Autodesk Fusion 360 part; units mm, degrees
sketch "Sketch1" plane through (0, 0, 0) normal (0, 0, 1) x (1, 0, 0)
  line L0 (-120.55, 25.4) -> (120.65, 25.4)
  line L1 (120.65, 25.4) -> (120.65, -25.4)
  line L2 (120.65, -25.4) -> (-120.55, -25.4)
  line L3 (-120.55, -25.4) -> (-120.55, 25.4)
  dimension "d3" = 241.2
  dimension "d4" = 50.8
  dimension "d5" = 25.4
  dimension "d6" = 120.65
extrude "Extrude1" add sketch "Sketch1" along normal blind 2.5
sketch "Sketch2" plane through (0, 0, 2.5) normal (0, 0, 1) x (-1, 0, 0)
  line L0 (120.55, 25.4) -> (-120.65, 25.4)
  line L1 (-120.65, 25.4) -> (-120.65, -25.4)
  line L2 (-120.65, -25.4) -> (120.55, -25.4)
  line L3 (120.55, -25.4) -> (120.55, 25.4)
  line L4 (13.4, -15.4) -> (-13.4, -15.4)
  line L5 (-15.4, -13.4) -> (-15.4, 13.4)
  line L6 (-13.4, 15.4) -> (13.4, 15.4)
  line L7 (15.4, 13.4) -> (15.4, -13.4)
  arc A0 (13.4, -15.4) -> (15.4, -13.4) centre (13.4, -13.4) ccw
  arc A1 (-15.4, -13.4) -> (-13.4, -15.4) centre (-13.4, -13.4) ccw
  arc A2 (-13.4, 15.4) -> (-15.4, 13.4) centre (-13.4, 13.4) ccw
  arc A3 (15.4, 13.4) -> (13.4, 15.4) centre (13.4, 13.4) ccw
  dimension "d7" = 30.8
  dimension "d8" = 30.8
  dimension "d9" = 15.4
  dimension "d10" = 15.4
  dimension "d11" = 2
extrude "Extrude2" cut sketch "Sketch2" against normal blind 2.5 contours L4 L5 L6 L7 A0 A1 A2 A3
sketch "Sketch4" plane through (0, 0, 2.5) normal (0, 0, 1) x (-1, 0, 0)
  line L0 (15.4, 13.4) -> (15.4, -13.4)
  arc A0 (13.4, -15.4) -> (15.4, -13.4) centre (13.4, -13.4) ccw
  line L1 (13.4, -15.4) -> (-13.4, -15.4)
  arc A1 (-15.4, -13.4) -> (-13.4, -15.4) centre (-13.4, -13.4) ccw
  line L2 (-15.4, -13.4) -> (-15.4, 13.4)
  arc A2 (-13.4, 15.4) -> (-15.4, 13.4) centre (-13.4, 13.4) ccw
  line L3 (-13.4, 15.4) -> (13.4, 15.4)
  arc A3 (15.4, 13.4) -> (13.4, 15.4) centre (13.4, 13.4) ccw
  line L4 (120.55, 25.4) -> (-120.65, 25.4)
  line L5 (-120.65, 25.4) -> (-120.65, -25.4)
  line L6 (-120.65, -25.4) -> (120.55, -25.4)
  line L7 (120.55, -25.4) -> (120.55, 25.4)
  line L8 (18, -20) -> (-18, -20)
  line L9 (-20, -18) -> (-20, 18)
  line L10 (-18, 20) -> (18, 20)
  line L11 (20, 18) -> (20, -18)
  arc A4 (18, -20) -> (20, -18) centre (18, -18) ccw
  arc A5 (-20, -18) -> (-18, -20) centre (-18, -18) ccw
  arc A6 (-18, 20) -> (-20, 18) centre (-18, 18) ccw
  arc A7 (20, 18) -> (18, 20) centre (18, 18) ccw
  dimension "d18" = 40
  dimension "d19" = 40
  dimension "d20" = 20
  dimension "d21" = 20
  dimension "d22" = 2
extrude "Extrude3" add sketch "Sketch4" along normal blind 2.5 contours L8 L9 L10 L11 A4 A5 A6 A7
sketch "Sketch6" plane through (0, 0, 5) normal (0, 0, 1) x (-1, 0, 0)
  arc A0 (13.4, -15.4) -> (15.4, -13.4) centre (13.4, -13.4) ccw
  line L0 (13.4, -15.4) -> (-13.4, -15.4)
  arc A1 (-15.4, -13.4) -> (-13.4, -15.4) centre (-13.4, -13.4) ccw
  line L1 (-15.4, -13.4) -> (-15.4, 13.4)
  arc A2 (-13.4, 15.4) -> (-15.4, 13.4) centre (-13.4, 13.4) ccw
  line L2 (-13.4, 15.4) -> (13.4, 15.4)
  arc A3 (15.4, 13.4) -> (13.4, 15.4) centre (13.4, 13.4) ccw
  line L3 (15.4, 13.4) -> (15.4, -13.4)
  arc A4 (18, -20) -> (20, -18) centre (18, -18) ccw
  line L4 (20, -18) -> (20, 18)
  arc A5 (20, 18) -> (18, 20) centre (18, 18) ccw
  line L5 (18, 20) -> (-18, 20)
  arc A6 (-18, 20) -> (-20, 18) centre (-18, 18) ccw
  line L6 (-20, 18) -> (-20, -18)
  arc A7 (-20, -18) -> (-18, -20) centre (-18, -18) ccw
  line L7 (-18, -20) -> (18, -20)
  point P0 (17, -17)
  point P1 (-17, -17)
  point P2 (-17, 17)
  point P3 (17, 17)
  dimension "d29" = 34
  dimension "d30" = 34
  dimension "d31" = 17
  dimension "d32" = 17
hole "Hole1" at (-17, 17, 5) at (17, 17, 5) at (17, -17, 5) at (-17, -17, 5) direction (0, 0, -1) diameter 2.54 depth 5 tip angle 118
chamfer "Chamfer1" distance 2.5 distance2 2.5 8 edges at (0, -20, 2.5) (-19.4142, -19.4142, 2.5) (-20, 0, 2.5) (-19.4142, 19.4142, 2.5) (0, 20, 2.5) (19.4142, 19.4142, 2.5) (20, 0, 2.5) (19.4142, -19.4142, 2.5) measured on face at (87.1, -6, 2.5) measured on face at (87.1, -6, 2.5) measured on face at (87.1, -6, 2.5) measured on face at (87.1, -6, 2.5) measured on face at (87.1, -6, 2.5) measured on face at (87.1, -6, 2.5) measured on face at (87.1, -6, 2.5) measured on face at (87.1, -6, 2.5)
fillet "Fillet1" radius 2.5 8 edges at (22.5, 0, 2.5) (21.182, 21.182, 2.5) (0, 22.5, 2.5) (-21.182, 21.182, 2.5) (-22.5, 0, 2.5) (-21.182, -21.182, 2.5) (0, -22.5, 2.5) (21.182, -21.182, 2.5)
sketch "Sketch7" plane through (0, 0, 0) normal (0, 0, -1) x (1, 0, 0)
  circle A0 centre (17, 17) radius 1.27
  circle A1 centre (-17, -17) radius 1.27
  circle A2 centre (17, -17) radius 1.27
  circle A3 centre (-17, 17) radius 1.27
  line L0 (-15.4, -13.4) -> (-15.4, 13.4)
  arc A4 (-13.4, 15.4) -> (-15.4, 13.4) centre (-13.4, 13.4) ccw
  line L1 (-13.4, 15.4) -> (13.4, 15.4)
  arc A5 (15.4, 13.4) -> (13.4, 15.4) centre (13.4, 13.4) ccw
  line L2 (15.4, 13.4) -> (15.4, -13.4)
  arc A6 (13.4, -15.4) -> (15.4, -13.4) centre (13.4, -13.4) ccw
  line L3 (13.4, -15.4) -> (-13.4, -15.4)
  arc A7 (-15.4, -13.4) -> (-13.4, -15.4) centre (-13.4, -13.4) ccw
  line L4 (120.65, 25.4) -> (-120.55, 25.4)
  line L5 (-120.55, 25.4) -> (-120.55, -25.4)
  line L6 (-120.55, -25.4) -> (120.65, -25.4)
  line L7 (120.65, -25.4) -> (120.65, 25.4)
  point P0 (-112.9, 15)
  point P1 (-112.9, -15)
  point P2 (113, 15)
  point P3 (113, -15)
  dimension "d40" = 30
  dimension "d41" = 7.65
  dimension "d42" = 7.65
  dimension "d48" = 10.4
hole "Hole2" at (-112.9, -15, 0) at (-112.9, 15, 0) at (113, -15, 0) at (113, 15, 0) direction (0, 0, 1) diameter 4.5 depth 5 tip angle 180 countersink diameter 9.4 countersink angle 90
extrude "Extrude5" add 1 faces at (-17.0425, 4.4667, 5) along direction (0, 0, 1) blind 10
equation "d3 = 9.5 in - 0.1 mm"
equation "d6 = ( 9.5 / 2 ) * 1 in"
equation "d41 = ( ( 15.4 / 2 ) * 1 mm ) - 0.05 * 1 mm"
equation "d42 = ( ( 15.4 / 2 ) * 1 mm ) - 0.05 * 1 mm"
equation "d48 = ( 2 in - 30 mm ) / 2"
Input: part model. Units: mm. Frame: model coordinates. A direction names the side the tool comes from. Give positions to 0.01 mm unless a question says otherwise; leave off trailing zeros. Write each loop counter-clockwise with the first axis right and the second up, starting at its lowest first coordinate (ties: lowest second). Pieces come first, ordered by that corner, then holes. Notation, with made-up numbers: (-6, 74.5) - (27, 74.5) arc R16 ccw to (27, 82.5) - close; hole circle Ø1 at (13.25, -33). An arc over 180 degrees is marked (long way). Write item = value, one per line. Start each with the question number.
1) Cut plane D-D (x = -42). Return loops of the section in (y, z).
2) Reachability of faces 4 (the face through (20, 0, 10)), 5 (the face through (0, -20, 10)), 6 (the face through (0, 15.4, 7)) from +Z, -Z, +X, -X, +Y, -Y: full face, straight path, thin tool, end or side. Return the list, or none.
3) Draft query along X for faces 1 (the face through (-20, 0, 10)), 2 (the face through (0, 20, 10)), 3 (the face through (-15.4, 0, 7)). Return one class per face: pulls with the +X half, pulls with the -X half, needs draft (parallel to the pull), parting line crosses it, or undercut.
4) Cut plane C-C (y = -3). Return loops of the section in (x, z).
5) Cut plane A-A (x = -112.9). Return loops of the section in (y, z), and give its area (3 significant figures).
6) Material intervals for L1, parallel to X at y = -17, z = 8; L2, parallel to Y at x = -4, z = 6.5, sorted ascending. Write a range as [from, to].
7) Cut plane B-B (z = 8.5). Return loops of the section in (x, y), and give its area (3 significant figures).
8) Pin query (flat end, axial travel): pin 1 (4 mm diameter, centred on x = -17, y = 17, fed in from +Z); pin 2 (5 mm diameter, centred on x = -8.5, z = 9, fed in from -Y); pin 3 (5 mm diameter, centred on x = -112.9, y = -15, fed in from -Z); pin 4 (1.5 mm diameter, centred on y = -12, z = 5, fed in from +X). Return the tip coordinate at first contact, or that it passes through.
Answers follow:
q1.outline = (-25.4, 0) - (25.4, 0) - (25.4, 2.5) - (-25.4, 2.5) - close
q2.face_4 = +Z, +X, +Y, -Y
q2.face_5 = +Z, +X, -X, -Y
q2.face_6 = +Z, -Z
q3.face_1 = pulls with the -X half
q3.face_2 = needs draft
q3.face_3 = undercut
q4.outline = (-120.55, 0) - (-15.4, 0) - (-15.4, 15) - (-20, 15) - (-20, 5) - (-21.77, 3.23) arc R2.5 cw to (-23.54, 2.5) - (-120.55, 2.5) - close; (15.4, 0) - (120.65, 0) - (120.65, 2.5) - (23.54, 2.5) arc R2.5 cw to (21.77, 3.23) - (20, 5) - (20, 15) - (15.4, 15) - close
q5.outline = (-25.4, 0) - (-19.7, 0) - (-17.25, 2.45) - (-17.25, 2.5) - (-25.4, 2.5) - close; (-12.75, 2.45) - (-10.3, 0) - (10.3, 0) - (12.75, 2.45) - (12.75, 2.5) - (-12.75, 2.5) - close; (17.25, 2.45) - (19.7, 0) - (25.4, 0) - (25.4, 2.5) - (17.25, 2.5) - close
q5.area = 92.5 mm^2
q6.L1 = [-20, -18.27], [-15.73, 15.73], [18.27, 20]
q6.L2 = [-20, -15.4], [15.4, 20]
q7.outline = (-20, -18) arc R2 ccw to (-18, -20) - (18, -20) arc R2 ccw to (20, -18) - (20, 18) arc R2 ccw to (18, 20) - (-18, 20) arc R2 ccw to (-20, 18) - close; hole circle Ø2.54 at (-17, -17); hole circle Ø2.54 at (-17, 17); hole (-15.4, -13.4) arc R2 ccw to (-13.4, -15.4) - (13.4, -15.4) arc R2 ccw to (15.4, -13.4) - (15.4, 13.4) arc R2 ccw to (13.4, 15.4) - (-13.4, 15.4) arc R2 ccw to (-15.4, 13.4) - close; hole circle Ø2.54 at (17, -17); hole circle Ø2.54 at (17, 17)
q7.area = 631 mm^2
q8.pin_1 = 15
q8.pin_2 = -20
q8.pin_3 = 2.2
q8.pin_4 = 20.75
